Verification items for the finished model (mm, model axes). A direction names the side the tool comes from. Round coordinates to 2 decimals unless told otherwise and drop trailing zeros. Write each loop counter-clockwise with the first axis right and the second up, starting at its lowest first coordinate (ties: lowest second). Pieces come first, ordered by that corner, then holes. Notation, with made-up numbers: (67.5, -36) - (74.5, -36) arc R26 ccw to (74.5, -20) - close; hole circle Ø1 at (5, 57.5). An arc over 180 degrees is marked (long way). Answer as a JSON object with one key per item and string values.
Autodesk Inventor part; units mm, degrees
ref_plane "YZ Plane" through (0, 0, 0) normal (1, 0, 0) x (0, 1, 0)
ref_plane "XZ Plane" through (0, 0, 0) normal (0, 1, 0) x (-1, 0, 0)
ref_plane "XY Plane" through (0, 0, 0) normal (0, 0, 1) x (1, 0, 0)
sketch "Sketch1" plane through (0, 0, 0) normal (0, 0, 1) x (1, 0, 0)
  line L0 (0, 0) -> (100, 0)
  line L1 (100, 0) -> (100, 500)
  line L2 (100, 500) -> (0, 500)
  line L3 (0, 500) -> (0, 0)
  dimension "d0" = 100
  dimension "d1" = 500
extrude "Extrusion1" add sketch "Sketch1" along normal blind 40
sketch "Sketch2" plane through (0, 0, 40) normal (0, 0, 1) x (1, 0, 0)
  line L0 (0, 0) -> (100, 0)
  line L1 (50, 0) -> (50, 10)
  dimension "d4" = 10
sketch "Sketch3" plane through (0, 0, 40) normal (0, 0, 1) x (1, 0, 0)
  line L0 (100, 500) -> (0, 500)
  line L1 (50, 500) -> (50, 490)
  line L2 (100, 0) -> (100, 500)
  line L3 (100, 250) -> (90, 250)
  line L4 (0, 500) -> (0, 0)
  line L5 (0, 250) -> (10, 250)
  line L6 (90, 490) -> (10, 490)
  line L7 (10, 490) -> (10, 9.7366)
  line L8 (10, 9.7366) -> (90, 9.7366)
  line L9 (90, 9.7366) -> (90, 490)
  dimension "d5" = 10
  dimension "d7" = 10
extrude "Extrusion2" cut sketch "Sketch3" against normal blind 30 contours L6 L9 L8 L7
properties part number "S.hollow box"
1. Cross-section at C-C (y = 40). Record the boundary of the cut face in (x, z).
Completed:
{"outline": "(0, 0) - (100, 0) - (100, 40) - (90, 40) - (90, 10) - (10, 10) - (10, 40) - (0, 40) - close"}
2. Mould release check, pull along Y, two halves, no side actions. Record for faces 1 (the face through (0, 253, 20)), 2 (the face through (90, 247, 25)), 3 (the face through (49, 0, 20)): released by +Y, released by -Y, zero draft, split by the parting line, or undercut.
Completed:
{"face 1": "zero draft", "face 2": "undercut", "face 3": "released by -Y"}
3. Access from +Z, -Z, +X, -X, +Y, -Y to the whole of each face (thin tool, end or side, straight path). Record for faces 4 (the face through (49, 254, 0)), 5 (the face through (49, 9.737, 25)).
Completed:
{"face 4": "-Z, +X, -X, +Y, -Y", "face 5": "+Z"}
4. Material ranges on probe 1 along Y at (x, z) = (76, 28.5); probe 2 along X at (y, z) = (66.5, 35); probe 3 along Z at (x, y) = (12, 42.5), recorded low to high. Write a range as from..to.
Completed:
{"probe 1": "y = 0..9.74, 490..500", "probe 2": "x = 0..10, 90..100", "probe 3": "z = 0..10"}
5. Go/stop test with flat-tipped pins: pin 1 (15 mm diameter, centred on x = 52, z = 30, fed in from -Y); pin 2 (12 mm diameter, centred on x = 26.5, y = 403.5, fed in from +Z). Record where each tip stops, or that it passes through.
Completed:
{"pin 1": "stops at y = 0", "pin 2": "stops at z = 10"}
6. Cross-section at A-A (z = 23.5). Record the boundary of the cut face in (x, y).
Completed:
{"outline": "(0, 0) - (100, 0) - (100, 500) - (0, 500) - close; hole (10, 9.74) - (90, 9.74) - (90, 490) - (10, 490) - close"}
7. Cross-section at B-B (x = 34). Record the boundary of the cut face in (y, z).
Completed:
{"outline": "(0, 0) - (500, 0) - (500, 40) - (490, 40) - (490, 10) - (9.74, 10) - (9.74, 40) - (0, 40) - close"}
